from build123d import *

# Parameters (mm, degrees)
BOSS_EXTRUDE1_DEPTH = 10
SKETCH2_W           = 1.866494487
SKETCH2_H           = 2.78
SKETCH2_H_2         = 1
BOSS_EXTRUDE2_DEPTH = 1
BOSS_EXTRUDE3_DEPTH = 3
SKETCH4_W           = 14.931955898
SKETCH4_H           = 1
BOSS_EXTRUDE4_DEPTH = 1
SKETCH5_W           = 14.931955898
SKETCH5_H           = 0.998682686
BOSS_EXTRUDE5_DEPTH = 1
CUT_EXTRUDE1_DEPTH  = 15
CUT_EXTRUDE2_DEPTH  = 15
CUT_EXTRUDE3_DEPTH  = 15


with BuildPart() as part:
    # Sketch1 → Boss-Extrude1 (new body)
    with BuildSketch(Plane(origin=(0, 0, 0), x_dir=(1, 0, 0), z_dir=(0, 1, 0))):
        Polygon((-13.931955898, 6.56), (-13.931955898, -1), (-13, -1), (-13, 0), (-13, 5.56), (0, 5.56), (0, 0), (1, 0), (1, 5.56), (1, 6.56), (-12.931955898, 6.56), align=None)
        Polygon((0, -1), (1, -1), (1, 0), (0, 0), (-13, 0), (-13, -1), align=None)
    extrude(amount=BOSS_EXTRUDE1_DEPTH)

    # Sketch2 → Boss-Extrude2 (add)
    with BuildSketch(Plane(origin=(0, 10, 0), x_dir=(1, 0, 0), z_dir=(0, 1, 0))):
        Polygon((-13, 0), (-6.465977949, 0), (-6.465977949, 2.78), (-6.465977949, 5.56), (-13, 5.56), align=None)
        with Locations((-5.532730706, 4.17)):
            Rectangle(SKETCH2_W, SKETCH2_H)
        with Locations((-5.532730706, 1.39)):
            Rectangle(SKETCH2_W, SKETCH2_H)
        Polygon((-13.931955898, -1), (-6.465977949, -1), (-6.465977949, 0), (-13, 0), (-13, 5.56), (-6.465977949, 5.56), (-6.465977949, 6.56), (-13.931955898, 6.56), align=None)
        with Locations((-5.532730706, -0.5)):
            Rectangle(SKETCH2_W, SKETCH2_H_2)
        with Locations((-5.532730706, 6.06)):
            Rectangle(SKETCH2_W, SKETCH2_H_2)
    extrude(amount=-BOSS_EXTRUDE2_DEPTH)

    # Sketch3 → Boss-Extrude3 (add)
    with BuildSketch(Plane(origin=(0, 10, 0), x_dir=(1, 0, 0), z_dir=(0, 1, 0))):
        Polygon((1, 6.56), (-12.931955898, 6.56), (-12.931955898, 5.56), (-4.599483462, 5.56), (0, 5.56), (0, 0), (-4.599483462, 0), (-12.931955898, 0), (-12.931955898, -1), (1, -1), align=None)
        Polygon((-12.931955898, 6.56), (-13.931955898, 6.56), (-13.931955898, -1), (-12.931955898, -1), (-12.931955898, 0), (-12.931955898, 5.56), align=None)
    extrude(amount=BOSS_EXTRUDE3_DEPTH)

    # Sketch4 → Boss-Extrude4 (add)
    with BuildSketch(Plane.XY.offset(1)):
        with Locations((-6.465977949, 12.5)):
            Rectangle(SKETCH4_W, SKETCH4_H)
    extrude(amount=BOSS_EXTRUDE4_DEPTH)

    # Sketch5 → Boss-Extrude5 (add)
    with BuildSketch(Plane(origin=(0, 0, -6.56), x_dir=(-1, 0, 0), z_dir=(0, 0, -1))):
        with Locations((6.465977949, 12.500658657)):
            Rectangle(SKETCH5_W, SKETCH5_H)
    extrude(amount=BOSS_EXTRUDE5_DEPTH)

    # Sketch6 → Cut-Extrude1 (cut)
    with BuildSketch(Plane.ZY.offset(13.931955898)):
        Polygon((-7.56, 12.001317314), (-6.56, 13), (-7.56, 13), align=None)
        Polygon((1, 13), (2, 12), (2, 13), align=None)
    extrude(amount=-CUT_EXTRUDE1_DEPTH, mode=Mode.SUBTRACT)

    # Sketch7 → Cut-Extrude2 (cut)
    with BuildSketch(Plane(origin=(1, 0, 0), x_dir=(0, 0, -1), z_dir=(1, 0, 0))):
        Polygon((-1.5, 12), (-1, 13), (-2, 12), align=None)
        Polygon((7.56, 12.001317314), (6.56, 13), (7.06, 12.001317314), align=None)
    extrude(amount=-CUT_EXTRUDE2_DEPTH, mode=Mode.SUBTRACT)

    # Sketch12 → Cut-Extrude3 (cut)
    with BuildSketch(Plane.ZY.offset(13.931955898)):
        Polygon((-6.81, 12.500658657), (-6.56, 12.500658657), (-6.56, 13), align=None)
        Polygon((-6.56, 13), (-6.56, 12.500658657), (-5.56, 13), align=None)
        Polygon((1.25, 12.5), (1, 13), (1, 12.5), align=None)
        Polygon((1, 12.5), (1, 13), (0, 13), align=None)
    extrude(amount=-CUT_EXTRUDE3_DEPTH, mode=Mode.SUBTRACT)


solid = part.part
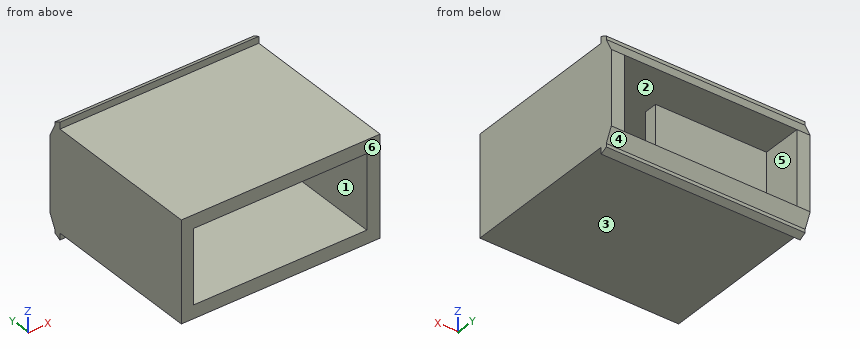
Verification items for the finished model (mm, model axes). Face numbers are marked on the shaded views. A direction names the side the tool comes from. Coordinates: 2 decimals unless noted, no trailing zeros. Write each loop counter-clockwise with the first axis right and the second up, starting at its lowest first coordinate (ties: lowest second). Pieces come first, ordered by that corner, then holes. Notation, with made-up numbers: M 54,60.5 L 95,60.5 A19 cw 95,83.5 Z; hole C 56.25,7.5 d3. An arc over 180 degrees is marked long. Use CSV: the item, a comma, the result in double quotes.
Q1. Thickness scan on line 1 along Z through (x, y) = (-6.75, 7); line 2 along X through (y, z) = (7.75, -1.25); line 3 along X through (y, z) = (11.75, -1.5). Record the ranges inside material, lowest first. Write a range as [from, to].
Computed values:
line 1,"[-6.56, -5.56], [0, 1]"
line 2,"[-13.93, -13], [0, 1]"
line 3,"[-13.93, -12.93], [0, 1]"
Q2. Section check A-A, the plane x = -3. Enter the section's corners in (y, z), and give its area (3 significant figures).
Computed values:
outline,"M 0,-6.56 L 12,-6.56 L 12,-7.06 L 12.5,-6.81 L 12.5,-6.56 L 13,-5.56 L 0,-5.56 Z; M 0,0 L 13,0 L 12.5,1 L 12.5,1.25 L 12,1.5 L 12,1 L 0,1 Z"
area,"25.9 mm²"
Q3. Section check C-C, the plane y = 12.25. Enter the section's corners in (x, z) (1 decimal).
Computed values:
outline,"M -13.9,-6.9 L 1,-6.9 L 1,1.4 L -13.9,1.4 Z; hole M -12.9,-5.6 L 0,-5.6 L 0,0 L -12.9,0 Z"
Q4. Section check B-B, the plane z = -3. Enter the section's corners in (x, y), and give its area (3 significant figures).
Computed values:
outline,"M -13.93,0 L -13,0 L -13,9 L -4.6,9 L -4.6,10 L -12.93,10 L -12.93,13 L -13.93,13 Z; M 0,0 L 1,0 L 1,13 L 0,13 Z"
area,"33.7 mm²"
Q5. Mould release check, pull along Z, two halves, no side actions. Record for the marked faces 4, 5 and 6: pulls with the +Z half, pulls with the -Z half, needs draft (parallel to the pull), parting line crosses it, or undercut.
Computed values:
face 4,"pulls with the -Z half"
face 5,"undercut"
face 6,"needs draft"
Q6. Go/stop test with flat-tipped pins: P1, Ø3, axis at x = -8.5, z = -2, coming from the +Y side; P2, Ø1.5, axis at x = -1, y = 6.5, coming from the -Z side; P3, Ø1.7, axis at x = -9.5, z = -3, coming from the -Y side. Record where each tip stops, or that it passes through.
Computed values:
P1,"y = 10"
P2,"z = -6.56"
P3,"y = 9"
Q7. Set-up check for the marked faces 1, 2 and 3: record each of +Z, -Z, +X, -X, +Y, -Y from which the full face is reachable in a straight line by a thin tool's end or side.
Computed values:
face 1,"+Y, -Y"
face 2,"none"
face 3,"-Z, +X, -X, -Y"
Q8. Section check D-D, the plane x = -9.25. Enter the section's corners in (y, z).
Computed values:
outline,"M 0,-6.56 L 12,-6.56 L 12,-7.06 L 12.5,-6.81 L 12.5,-6.56 L 13,-5.56 L 10,-5.56 L 10,0 L 13,0 L 12.5,1 L 12.5,1.25 L 12,1.5 L 12,1 L 0,1 L 0,0 L 9,0 L 9,-5.56 L 0,-5.56 Z"
